Could you check a few things on this drawing? It's one solid part, dimensions in mm from its lowest x, y, z. Give positions to 0.01 mm unless a question says otherwise; leave off trailing zeros. Order: outer loops, then holes, each group sorted by start corner. A loop starts at its lowest first (then second) coordinate and runs counter-clockwise, first axis right, second up.
Item 1: I want a section at C-C, the plane z = 6. Write out the boundary of the cut face in (x, y) (1 decimal).
Item 2: I want a section at A-A, the plane x = 33.5. Write out the boundary of the cut face in (y, z).
Item 3: If I drill on line 1 along Z through (x, y) = (10, 1.4); line 2 along X through (y, z) = (1.65, 10); line 3 along X through (y, z) = (4.3, 14.5) (1 decimal), over which ranges is the centre line in solid material (lowest first)?
Item 4: If we mould it in two halves opening along X, with no side actions, what happens to the marked faces 1 and 2? For each: +X half, -X half, draft (parallel to the pull), parting line (faces both ways), or undercut.
Item 5: I want a section at B-B, the plane y = 3.7. Count the separate pieces of the cut face and the enclosed holes in it, then the cut area to 3 significant figures.
Item 6: I'm going to push flat-ended pins straight in: pin 1 Ø1 at (x, y) = (26, 4.5) entering from -Z; pin 2 Ø1.5 at (x, y) = (26, 1) entering from -Z; pin 3 Ø1 at (x, y) = (33.5, 4) entering from +Z; pin 4 Ø7 at (x, z) = (31.5, 8.5) entering from -Y. Where does each tip first touch, or does it pass through?
Item 7: I want a section at D-D, the plane x = 10. Write out the boundary of the cut face in (y, z).
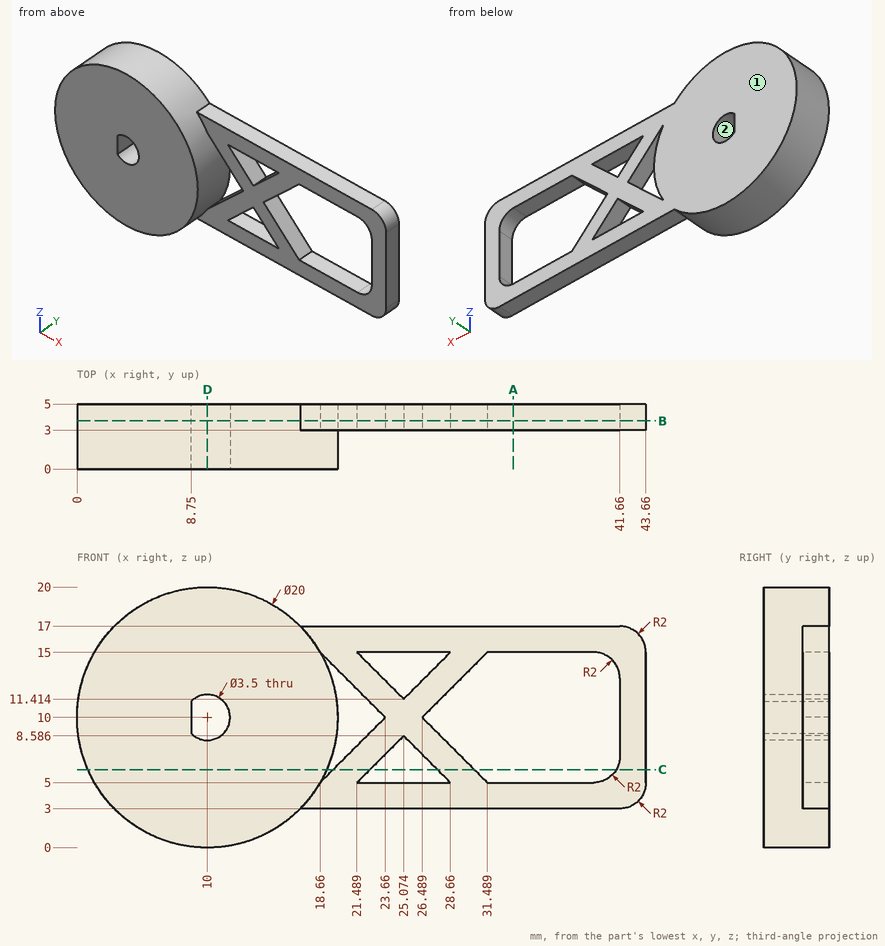
Results list:
1. outline: (0.8, 0) - (19.2, 0) - (19.2, 5) - (0.8, 5) - close; (19.7, 3) - (22.5, 3) - (22.5, 5) - (19.7, 5) - close; (27.7, 3) - (30.5, 3) - (30.5, 5) - (27.7, 5) - close; (41.4, 3) - (43.7, 3) - (43.7, 5) - (41.4, 5) - close
2. outline: (3, 3) - (5, 3) - (5, 5) - (3, 5) - close; (3, 15) - (5, 15) - (5, 17) - (3, 17) - close
3. line 1: z = 0 to 8.25, 11.75 to 20
3. line 2: x = 0 to 8.75, 11.75 to 20
3. line 3: x = 1.1 to 18.9, 19.2 to 22, 28.2 to 31, 41 to 43.7
4. face 1: draft
4. face 2: undercut
5. separate pieces: 1
5. enclosed holes: 5
5. area: 481 mm2
6. pin 1: stops at z = 3
6. pin 2: passes through
6. pin 3: stops at z = 17
6. pin 4: stops at y = 3
7. outline: (0, 0) - (5, 0) - (5, 8.25) - (0, 8.25) - close; (0, 11.75) - (5, 11.75) - (5, 20) - (0, 20) - close
